For this review, take the finished solid that the model builds, in its own axes (mm). A direction names the side the tool comes from. Round coordinates to 2 decimals unless told otherwise and drop trailing zeros. Order: outer loops, then holes, each group sorted by start corner. A loop starts at its lowest first (then second) coordinate and runs counter-clockwise, first axis right, second up. Notation, with made-up numbers: M 50,-9.5 L 55,-9.5 A27 ccw 55,29.5 Z; hole C -34,74 d10. An arc over 180 degrees is marked long. Answer as a JSON object with one key per item and string values.
Autodesk Fusion 360 part; units mm, degrees
sketch "Sketch1" plane through (0, 0, 0) normal (0, 0, 1) x (1, 0, 0) in component "RadPad"
  line L0 (-23, 0) -> (67.25, 0)
  line L1 (69.25, -2) -> (69.25, -93.25)
  line L2 (67.25, -95.25) -> (-5, -95.25)
  line L3 (-25, -75.25) -> (-25, -2)
  line L4 (-32.5, 9.5) -> (77.75, 9.5)
  line L5 (79.75, 7.5) -> (79.75, -103.75)
  line L6 (77.75, -105.75) -> (-8, -105.75)
  line L7 (-34.5, -79.25) -> (-34.5, 7.5)
  circle A0 centre (-17.8395, -88.8395) radius 1.7
  circle A1 centre (74.75, -100.75) radius 1.7
  circle A2 centre (74.75, 4.5) radius 1.7
  circle A3 centre (-29.5, 4.5) radius 1.7
  circle A4 centre (-29.5, 4.5) radius 3
  circle A5 centre (74.75, 4.5) radius 3
  circle A6 centre (74.75, -100.75) radius 3
  circle A7 centre (-17.8395, -88.8395) radius 3
  line L8 (-25, -75.25) -> (-5, -95.25)
  line L9 (-34.5, -79.25) -> (-8, -105.75)
  line L10 (-32.5, 9.5) -> (-34.5, 7.5)
  line L11 (-25, -2) -> (-23, 0)
  line L12 (67.25, 0) -> (69.25, -2)
  line L13 (69.25, -93.25) -> (67.25, -95.25)
  line L14 (79.75, -103.75) -> (77.75, -105.75)
  line L15 (77.75, 9.5) -> (79.75, 7.5)
  point P0 (-25, 0)
  point P1 (69.25, 0)
  point P2 (69.25, -95.25)
  point P3 (-25, -95.25)
  point P4 (-34.5, 9.5)
  point P5 (79.75, 9.5)
  point P6 (79.75, -105.75)
  point P7 (-34.5, -105.75)
  point P8 (75, -100)
  dimension "d1" = 94.25
  dimension "d2" = 95.25
  dimension "d3" = 114.25
  dimension "d4" = 115.25
  dimension "d5" = 9.5
  dimension "d6" = 9.5
  dimension "d7" = 3.4
  dimension "d8" = 3.4
  dimension "d9" = 3.4
  dimension "d10" = 3.4
  dimension "d11" = 5
  dimension "d12" = 5
  dimension "d15" = 5
  dimension "d16" = 5
  dimension "d17" = 5
  dimension "d18" = 5
  dimension "d19" = 6
  dimension "d20" = 6
  dimension "d21" = 6
  dimension "d22" = 6
  dimension "d23" = 20
  dimension "d24" = 20
  dimension "d25" = 26.5
  dimension "d26" = 26.5
  dimension "d27" = 5
  dimension "d28" = 2
  dimension "d29" = 2
  dimension "d30" = 2
  dimension "d31" = 2
  dimension "d32" = 2
  dimension "d33" = 2
  dimension "d34" = 2
  dimension "d35" = 2
  dimension "d36" = 2
  dimension "d37" = 2
  dimension "d38" = 2
  dimension "d39" = 2
extrude "Extrude1" add sketch "Sketch1" along normal blind 9.9 from surface at 3.1 contours A4 | A5 | A6 | A7 makes body 1 at (75.5625, 7.3879, 9.7) makes body 2 at (77.3099, -99.1857, 9.7) makes body 3 at (-26.5037, 4.3505, 9.7) makes body 4 at (-20.3993, -90.4038, 9.7) in component "RadPad"
extrude "Extrude2" add sketch "Sketch1" along normal blind 13 contours L4 L5 L6 L7 L9 L10 L14 L15 bodies 1 2 3 4 in component "RadPad"
extrude "Extrude3" add sketch "Sketch1" along normal blind 3 contours L0 L1 L2 L3 L8 L11 L12 L13 bodies 1 in component "RadPad"
sketch "Sketch2" plane through (0, 0, 13) normal (0, 0, 1) x (-1, 0, 0) in component "RadPad"
  circle A0 centre (-74.75, -4.5) radius 1.7
  circle A1 centre (17.8395, 88.8395) radius 1.7
  line L0 (5, 95.25) -> (25, 75.25)
  line L1 (25, 75.25) -> (25, 2)
  line L2 (25, 2) -> (23, 0)
  line L3 (23, 0) -> (-67.25, 0)
  line L4 (-67.25, 0) -> (-69.25, 2)
  line L5 (-69.25, 2) -> (-69.25, 93.25)
  line L6 (-69.25, 93.25) -> (-67.25, 95.25)
  line L7 (-67.25, 95.25) -> (5, 95.25)
  line L8 (32.5, -9.5) -> (34.5, -7.5)
  line L9 (34.5, -7.5) -> (34.5, 79.25)
  line L10 (34.5, 79.25) -> (8, 105.75)
  line L11 (8, 105.75) -> (-77.75, 105.75)
  line L12 (-77.75, 105.75) -> (-79.75, 103.75)
  line L13 (-79.75, 103.75) -> (-79.75, -7.5)
  line L14 (-79.75, -7.5) -> (-77.75, -9.5)
  line L15 (-77.75, -9.5) -> (32.5, -9.5)
  circle A2 centre (-74.75, 100.75) radius 1.7
  circle A3 centre (29.5, -4.5) radius 1.7
  line L16 (16.615, -9.5) -> (-1.885, -9.5)
  line L17 (-1.885, -9.5) -> (-1.885, 0)
  line L18 (-1.885, 0) -> (16.615, 0)
  line L19 (16.615, 0) -> (16.615, -9.5)
  line L20 (34.5, 79.25) -> (34.5, -7.5)
  point P0 (25, 0)
  dimension "d47" = 18.5
  dimension "d49" = 17.885
extrude "Extrude4" cut sketch "Sketch2" against normal blind 7.5 contours L3 L15 L16 L17 L18 L19 bodies 1 in component "RadPad"
component "RadPad" placed x (1, 0, 0) y (0, 1, 0) z (0, 0, 1) at (0, 0, 0)
equation "d24 = d23"
equation "d26 = d25"
equation "d29 = d28"
equation "d31 = d30"
equation "d33 = d32"
equation "d35 = d34"
equation "d37 = d36"
equation "d39 = d38"
equation "d49 = 12.135 mm + 5.75 mm"
1) Add section A-A on y = -100.75. State the section outline as (x, z) points.
Geometry check:
{"outline": "M -13,0 L 71.75,0 L 71.75,3.1 L 73.05,3.1 L 73.05,13 L -13,13 Z; M 76.45,3.1 L 77.75,3.1 L 77.75,0 L 79.75,0 L 79.75,13 L 76.45,13 Z"}
2) Add section D-D on x = 74.75. State the section outline as (y, z) points, and give its area (3 significant figures).
Geometry check:
{"outline": "M -105.75,0 L -103.75,0 L -103.75,3.1 L -102.45,3.1 L -102.45,13 L -105.75,13 Z; M -99.05,3.1 L -97.75,3.1 L -97.75,0 L 1.5,0 L 1.5,3.1 L 2.8,3.1 L 2.8,13 L -99.05,13 Z; M 6.2,3.1 L 7.5,3.1 L 7.5,0 L 9.5,0 L 9.5,13 L 6.2,13 Z", "area": "1,390 mm²"}
3) Add section B-B on x = -29.5. State the section outline as (y, z) points.
Geometry check:
{"outline": "M -84.25,0 L 1.5,0 L 1.5,3.1 L 2.8,3.1 L 2.8,13 L -84.25,13 Z; M 6.2,3.1 L 7.5,3.1 L 7.5,0 L 9.5,0 L 9.5,13 L 6.2,13 Z"}
4) Machinability: for faces 1 (the flat face through (-16.615, 5, 9)), 2 (the flat face through (32, 0, 8)), 3 (the flat face through (77, -101, 3.1)), which of the approach directions +Z, -Z, +X, -X, +Y, -Y give a long, thin tool a straight path to every point of the face, cutting with its end or side? Answer none if there is none.
Geometry check:
{"face 1": "+Z, +Y", "face 2": "+Z", "face 3": "-Z"}
5) Insertion check: P1, Ø2, axis at x = 74.75, y = 4.5, coming from the -Z side; P2, Ø1.5, axis at x = -15.5, y = -2, coming from the +Z side; P3, Ø3, axis at x = -10.5, y = 5.5, coming from the +Z side; P4, Ø1.8, axis at x = 73.5, y = -100, coming from the -Z side. Each pin has a flat end and moves straight along its axis. Give the tip position at first contact, or say it passes through.
Geometry check:
{"P1": "passes through", "P2": "stops at z = 3", "P3": "stops at z = 5.5", "P4": "stops at z = 3.1"}
6) Add section C-C on y = 4.5. State the section outline as (x, z) points (3 decimals).
Geometry check:
{"outline": "M -34.5,0 L -32.5,0 L -32.5,3.1 L -31.2,3.1 L -31.2,13 L -34.5,13 Z; M -27.8,3.1 L -26.5,3.1 L -26.5,0 L 71.75,0 L 71.75,3.1 L 73.05,3.1 L 73.05,13 L 1.885,13 L 1.885,5.5 L -16.615,5.5 L -16.615,13 L -27.8,13 Z; M 76.45,3.1 L 77.75,3.1 L 77.75,0 L 79.75,0 L 79.75,13 L 76.45,13 Z"}
7) Mouldability with a two-part tool opening along Y and no side actions: class faces 4 (the flat face through (-21.44, -92.31, 6.41)), 5 (the flat face through (-15.9, -88.8, 3.1)), 6 (the flat face through (-34.5, -36, 6)) as +Y half, -Y half, draft (parallel to the pull), parting line (faces both ways), or undercut.
Geometry check:
{"face 4": "-Y half", "face 5": "undercut", "face 6": "draft"}
8) For L1, parallel to Y at x = 74.75, z = 1.6; L2, parallel to Y at x = 74.75, z = 10.75; L3, parallel to X at y = -50.5, z = 10, list the stretches that pass through material, from the lowest coordinate up.
Geometry check:
{"L1": "y = -105.75 to -103.75, -97.75 to 1.5, 7.5 to 9.5", "L2": "y = -105.75 to -102.45, -99.05 to 2.8, 6.2 to 9.5", "L3": "x = -34.5 to -25, 69.25 to 79.75"}
